The model under review builds one solid part; all positions refer to its coordinate system, in mm. Round coordinates to 2 decimals unless told otherwise and drop trailing zeros. Order: outer loops, then holes, each group sorted by start corner. A loop starts at its lowest first (then second) coordinate and runs counter-clockwise, first axis right, second up. Notation, with made-up numbers: M -38,60.5 L -8,60.5 A27 ccw -8,91.5 Z; hole C 8,-0.75 d11. An arc over 180 degrees is marked long. Answer as a JSON object with one key per item and string values. Group by question number.
1. Add section A-A on x = 25.4. State the section outline as (y, z) points, and give its area (3 significant figures).
2. To check wall thickness, follow probe 1 along Y at (x, z) = (-25.4, -4.15); probe 2 along Y at (x, z) = (24, -4.5); probe 3 along X at (y, z) = (13.25, -4.5). State the ranges of each line that lie inside material, in increasing order. Write a range as [from, to].
3. Add section B-B on z = 1. State the section outline as (x, y) points (3 decimals), and give its area (3 significant figures).
4. Clearance check with flat-ended pins moving along their axes: P1, Ø1.1, axis at x = 6, y = -5.5, coming from the +Z side; P2, Ø2.5, axis at x = 25.4, y = 7.94, coming from the -Z side. State where each tip first meets the part, or that it passes through.
5. Add section C-C on y = -4.5. State the section outline as (x, z) points, and give its area (3 significant figures).
```python
from build123d import *

# Parameters (mm, degrees)
SKETCH1_W           = 62.738
SKETCH1_H           = 29.718
BOSS_EXTRUDE1_DEPTH = 5.08
FILLET1_R           = 2.54
SKETCH2_R           = 1.905
CUT_EXTRUDE1_DEPTH  = 5
SKETCH3_R           = 1.905
CUT_EXTRUDE2_DEPTH  = 3


with BuildPart() as part:
    # Sketch1 → Boss-Extrude1 (new body, symmetric)
    with BuildSketch(Plane.XY):
        Rectangle(SKETCH1_W, SKETCH1_H)
    extrude(amount=BOSS_EXTRUDE1_DEPTH, both=True)

    # Fillet1
    fillet1_edges = [part.edges().sort_by_distance(p)[0] for p in [
        (31.369, -14.859, 0),
        (-31.369, -14.859, 0),
        (-31.369, 14.859, 0),
        (31.369, 14.859, 0),
    ]]
    fillet(fillet1_edges, radius=FILLET1_R)

    # Sketch2 → Cut-Extrude1 (cut, symmetric)
    with BuildSketch(Plane.XY.offset(5.08)):
        with Locations((-5.7912, 5.715)):
            Circle(SKETCH2_R)
        with Locations((5.7912, 5.715)):
            Circle(SKETCH2_R)
        with Locations((5.7912, -5.715)):
            Circle(SKETCH2_R)
        with Locations((-5.7912, -5.715)):
            Circle(SKETCH2_R)
    extrude(amount=CUT_EXTRUDE1_DEPTH, both=True, mode=Mode.SUBTRACT)

    # Sketch3 → Cut-Extrude2 (cut, symmetric)
    with BuildSketch(Plane(origin=(0, 0, -5.08), x_dir=(-1, 0, 0), z_dir=(0, 0, -1))):
        with Locations((-25.4, 7.9375)):
            Circle(SKETCH3_R)
        with Locations((-25.4, -7.9375)):
            Circle(SKETCH3_R)
        with Locations((25.4, -7.9375)):
            Circle(SKETCH3_R)
        with Locations((25.4, 7.9375)):
            Circle(SKETCH3_R)
    extrude(amount=CUT_EXTRUDE2_DEPTH, both=True, mode=Mode.SUBTRACT)


solid = part.part
```
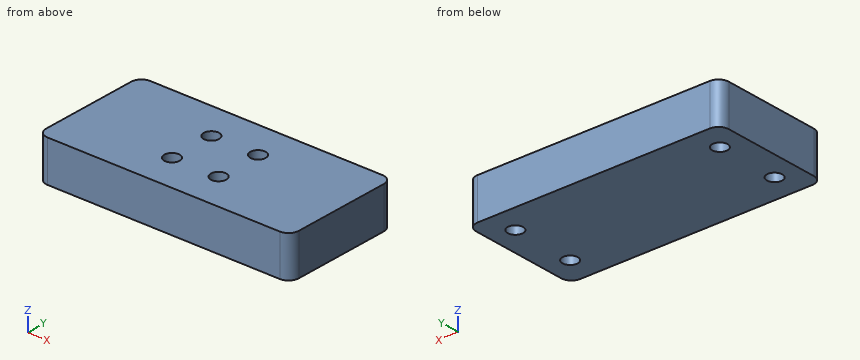
Recorded:
{
 "1": {"outline": "M -14.86,-5.08 L -9.84,-5.08 L -9.84,-2.08 L -6.03,-2.08 L -6.03,-5.08 L 6.03,-5.08 L 6.03,-2.08 L 9.84,-2.08 L 9.84,-5.08 L 14.86,-5.08 L 14.86,5.08 L -14.86,5.08 Z", "area": "279 mm²"},
 "2": {"probe 1": "y = [-14.86, -9.84], [-6.03, 6.03], [9.84, 14.86]", "probe 2": "y = [-14.86, -9.23], [-6.65, 6.65], [9.23, 14.86]", "probe 3": "x = [-31.19, 31.19]"},
 "3": {"outline": "M -31.369,-12.319 A2.54 ccw -28.829,-14.859 L 28.829,-14.859 A2.54 ccw 31.369,-12.319 L 31.369,12.319 A2.54 ccw 28.829,14.859 L -28.829,14.859 A2.54 ccw -31.369,12.319 Z; hole C -5.791,-5.715 d3.81; hole C -5.791,5.715 d3.81; hole C 5.791,-5.715 d3.81; hole C 5.791,5.715 d3.81", "area": "1,810 mm²"},
 "4": {"P1": "stops at z = 0.08", "P2": "stops at z = -2.08"},
 "5": {"outline": "M -31.37,-5.08 L 31.37,-5.08 L 31.37,5.08 L 7.26,5.08 L 7.26,0.08 L 4.32,0.08 L 4.32,5.08 L -4.32,5.08 L -4.32,0.08 L -7.26,0.08 L -7.26,5.08 L -31.37,5.08 Z", "area": "608 mm²"}
}
